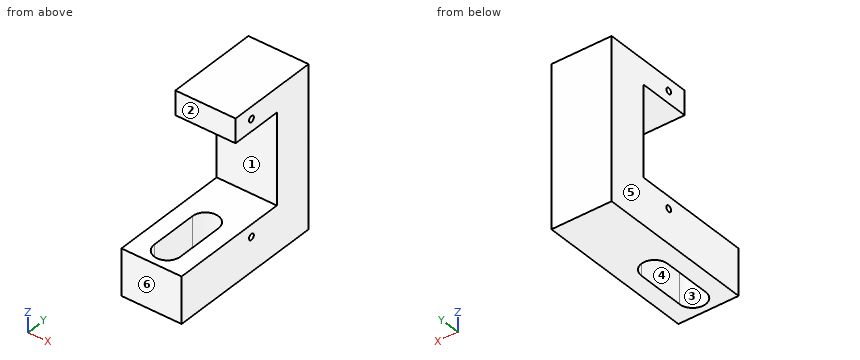
Autodesk Inventor part; units mm, degrees
ref_plane "YZ Plane" through (0, 0, 0) normal (1, 0, 0) x (0, 1, 0)
ref_plane "XZ Plane" through (0, 0, 0) normal (0, 1, 0) x (-1, 0, 0)
ref_plane "XY Plane" through (0, 0, 0) normal (0, 0, 1) x (1, 0, 0)
sketch "Sketch1" plane through (0, 0, 0) normal (1, 0, 0) x (0, 1, 0)
  line L0 (0, 0) -> (23, 0)
  line L1 (23, 0) -> (23, -40)
  line L2 (0, 0) -> (0, -6)
  line L3 (0, -6) -> (13, -6)
  line L4 (13, -6) -> (13, -28.5)
  line L5 (13, -28.5) -> (-17, -28.5)
  line L6 (23, -40) -> (-17, -40)
  line L7 (-17, -40) -> (-17, -28.5)
  circle A0 centre (5, -3) radius 0.75
  circle A1 centre (5, -31.5) radius 0.75
  point P0 (0, -3)
  dimension "d0" = 40
  dimension "d1" = 13
  dimension "d2" = 6
  dimension "d3" = 22.5
  dimension "d4" = 1.5
  dimension "d5" = 5
  dimension "d7" = 10
  dimension "d9" = 30
  dimension "d10" = 1.5
  dimension "d11" = 3
extrude "Extrusion1" add sketch "Sketch1" along normal blind 15
sketch "Sketch3" plane through (0, -17, -40) normal (0, 0, -1) x (-1, 0, 0)
  line L0 (-7.5, 17) -> (-7.5, 5) construction
  line L1 (-10.75, 17) -> (-10.75, 5)
  line L2 (-4.25, 5) -> (-4.25, 17)
  arc A0 (-4.25, 17) -> (-10.75, 17) centre (-7.5, 17) ccw
  arc A1 (-10.75, 5) -> (-4.25, 5) centre (-7.5, 5) ccw
  line L3 (0, 17) -> (-15, 17) construction
  point P0 (-7.5, 11)
  point P1 (-7.5, 17)
  dimension "d14" = 6.5
  dimension "d15" = 12
extrude "Extrusion2" cut sketch "Sketch3" against normal up to next
properties part number "servo mount"
CAD build for the part. Positions are in the model's coordinates, mm. Face numbers are marked on the shaded views. A direction names the side the tool comes from. Coordinates: 2 decimals unless noted, no trailing zeros. Order: outer loops, then holes, each group sorted by start corner. A loop starts at its lowest first (then second) coordinate and runs counter-clockwise, first axis right, second up. Notation, with made-up numbers: (-11.5, 41) -> (32.5, 41) arc R19 ccw to (32.5, 75) -> close; hole circle Ø4 at (57.5, -40). An arc over 180 degrees is marked (long way). Answer in a Markdown table with one row per item.
1) Which spindle directions (+Z, -Z, +X, -X, +Y, -Y) get a long thin tool onto all of the face, cutting with end or side? Do the marked faces 1, 2 and 3. Say none if no direction does.
Check values:
| item | result |
|---|---|
| face 1 | +X, -X, -Y |
| face 2 | +Z, +X, -X, -Y |
| face 3 | +Z, -Z |
2) Mould opens along X. For the marked faces 4, 5 and 6 say: pulls with the +X half, pulls with the -X half, needs draft (parallel to the pull), parting line crosses it, or undercut.
Check values:
| item | result |
|---|---|
| face 4 | undercut |
| face 5 | pulls with the -X half |
| face 6 | needs draft |
3) Band-saw the part on C-C (z = -31.5). List the corners of the cut face in (x, y), and give its area (3 significant figures).
Check values:
| item | result |
|---|---|
| outline | (0, -17) -> (15, -17) -> (15, 4.25) -> (0, 4.25) -> close; (0, 5.75) -> (15, 5.75) -> (15, 23) -> (0, 23) -> close; hole (4.25, -12) arc R3.25 ccw to (10.75, -12) -> (10.75, 0) arc R3.25 ccw to (4.25, 0) -> close |
| area | 466 mm2 |
4) Flat gauge pins, fed straight in: P1, Ø1.2, axis at y = 5, z = -31.5, coming from the +X side; P2, Ø7.5, axis at x = 7, z = -20.5, coming from the -Y side; P3, Ø1.8, axis at x = 9, z = -2.5, coming from the -Y side; P4, Ø8, axis at x = 9, y = -10, coming from the +Z side. Where does each tip first touch, or does it go through?
Check values:
| item | result |
|---|---|
| P1 | through |
| P2 | y = 13 |
| P3 | y = 0 |
| P4 | z = -28.5 |
5) Band-saw the part on B-B (y = 8). List the corners of the cut face in (x, z), and give its area (4 significant figures).
Check values:
| item | result |
|---|---|
| outline | (0, -40) -> (15, -40) -> (15, -28.5) -> (0, -28.5) -> close; (0, -6) -> (15, -6) -> (15, 0) -> (0, 0) -> close |
| area | 262.5 mm2 |
6) Band-saw the part on D-D (x = 13.75). List the corners of the cut face in (y, z).
Check values:
| item | result |
|---|---|
| outline | (-17, -40) -> (23, -40) -> (23, 0) -> (0, 0) -> (0, -6) -> (13, -6) -> (13, -28.5) -> (-17, -28.5) -> close; hole circle Ø1.5 at (5, -31.5); hole circle Ø1.5 at (5, -3) |
7) Band-saw the part on A-A (x = 7.5). List the corners of the cut face in (y, z), and give its area (3 significant figures).
Check values:
| item | result |
|---|---|
| outline | (-17, -40) -> (-15.25, -40) -> (-15.25, -28.5) -> (-17, -28.5) -> close; (0, -6) -> (13, -6) -> (13, -28.5) -> (3.25, -28.5) -> (3.25, -40) -> (23, -40) -> (23, 0) -> (0, 0) -> close; hole circle Ø1.5 at (5, -31.5); hole circle Ø1.5 at (5, -3) |
| area | 607 mm2 |
8) Drill centre lines: line 1 (Z direction, x = 3, y = 5); line 2 (X direction, y = -1, z = -37); line 3 (Z direction, x = 6, y = 6.5). Where is each one in solid material? Low to high.
Check values:
| item | result |
|---|---|
| line 1 | -40 to -32.25, -30.75 to -28.5, -6 to -3.75, -2.25 to 0 |
| line 2 | 0 to 4.25, 10.75 to 15 |
| line 3 | -40 to -28.5, -6 to 0 |
